The model under review builds one solid part; all positions refer to its coordinate system, in mm. Coordinates: 2 decimals unless noted, no trailing zeros. Loops run counter-clockwise (first coordinate to the right, second up) from the corner with the lowest first, then second, coordinate; pieces in that order, holes last. Notation, with made-up numbers: (13, 58) - (39, 58) arc R18 cw to (39, 87) - close; hole circle Ø6 at (41, 67). An arc over 180 degrees is marked (long way). Answer in a Markdown table with one row per item. Add a question column.
(1) For P1, Ø5, axis at y = -11.5, z = 544.5, coming from the -X side; P2, Ø10, axis at x = 9, y = 123.5, coming from the -Z side, all flat-tipped, find the tip position at first contact; note any pin that passes through.
(2) We need section A-A on y = 129. Write out the cut boundary in (x, z).
(3) For line 1 along Z through (x, y) = (19, 145.5); line 2 along Y through (x, z) = (4.75, 273.5), list the stretches that pass through material, from the lowest coordinate up.
(4) We need section C-C on x = 8.75. Write out the cut boundary in (y, z), plus the area to 3 significant figures.
(5) We need section B-B on z = 429. Write out the cut boundary in (x, y).
from build123d import *

# Parameters (mm, degrees)
SKETCH_W  = 580
SKETCH_H  = 166
PAD_DEPTH = 20


with BuildPart() as part:
    # Sketch → Pad (new body)
    with BuildSketch(Plane.YZ):
        Polygon((-290, 0), (-400, 0), (-400, 886), (400, 886), (400, 0), (290, 0), (290, 540), (-290, 540), align=None)
        with Locations((0, 703)):
            Rectangle(SKETCH_W, SKETCH_H, mode=Mode.SUBTRACT)
    extrude(amount=PAD_DEPTH)


solid = part.part
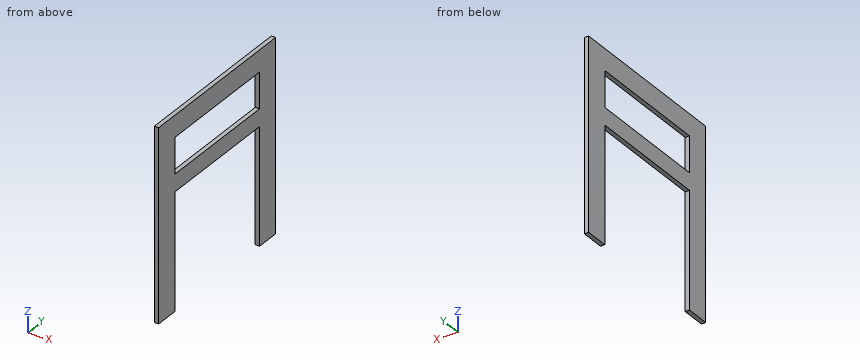
Outcome:
| question | item | result |
|---|---|---|
| 1 | P1 | x = 0 |
| 1 | P2 | z = 540 |
| 2 | outline | (0, 540) - (20, 540) - (20, 620) - (0, 620) - close; (0, 786) - (20, 786) - (20, 886) - (0, 886) - close |
| 3 | line 1 | 540 to 620, 786 to 886 |
| 3 | line 2 | -400 to -290, 290 to 400 |
| 4 | outline | (-400, 0) - (-290, 0) - (-290, 540) - (290, 540) - (290, 0) - (400, 0) - (400, 886) - (-400, 886) - close; hole (-290, 620) - (290, 620) - (290, 786) - (-290, 786) - close |
| 4 | area | 299,000 mm² |
| 5 | outline | (0, -400) - (20, -400) - (20, -290) - (0, -290) - close; (0, 290) - (20, 290) - (20, 400) - (0, 400) - close |
